Here's how the part is built. I have some questions about the finished solid (model axes, mm). A direction names the side the tool comes from. Coordinates: 2 decimals unless noted, no trailing zeros. Loops run counter-clockwise (first coordinate to the right, second up) from the corner with the lowest first, then second, coordinate; pieces in that order, holes last.
```python
from build123d import *

# Parameters (mm, degrees)
SKETCH1_W           = 15
SKETCH1_H           = 35
BOSS_EXTRUDE1_DEPTH = 5
SKETCH2_R           = 1
SKETCH2_W           = 12
SKETCH2_H           = 22
CUT_EXTRUDE1_DEPTH  = 5
BOSS_EXTRUDE2_DEPTH = 5


with BuildPart() as part:
    # Sketch1 → Boss-Extrude1 (new body)
    with BuildSketch(Plane.XY):
        with Locations((-15.154109589, 0.428082192)):
            Rectangle(SKETCH1_W, SKETCH1_H)
    extrude(amount=BOSS_EXTRUDE1_DEPTH)

    # Sketch2 → Cut-Extrude1 (cut)
    with BuildSketch(Plane.XY.offset(5)):
        with Locations((-15.154109589, -12.571917808)):
            Circle(SKETCH2_R)
        with Locations((-15.154109589, 13.428082192)):
            Circle(SKETCH2_R)
        with Locations((-15.154109589, 0.428082192)):
            Rectangle(SKETCH2_W, SKETCH2_H)
    extrude(amount=-CUT_EXTRUDE1_DEPTH, mode=Mode.SUBTRACT)

    # Sketch3 → Boss-Extrude2 (add)
    with BuildSketch(Plane.XY.offset(5)):
        Polygon((-22.654109589, -17.071917808), (-22.654109589, -30.804233772), (-20.282646179, -47.190952111), (-17.359431797, -56.865022466), (-13.811210888, -68.607486145), (0, -68.607486145), (6.832413717, -38.997592941), (-6.905605444, -30.804233772), (-7.654109589, -17.071917808), align=None)
    extrude(amount=-BOSS_EXTRUDE2_DEPTH)


solid = part.part
```
1. I need wall thicknesses on line 1 along X through (y, z) = (9.5, 2.35); line 2 along Y through (x, z) = (-12.5, 3.75); line 3 along X through (y, z) = (-14, 3.55). Which ranges of each line are inside material? Lowest first, please.
2. I want a section at A-A (y = 7). Please give me the cut outline in (x, z).
3. I want a section at C-C (z = 2.3). Please give me the cut outline in (x, y).
4. On a 3-axis mill with a long thin cutter (end or side, diameter ignored), from which of +Z, -Z, +X, -X, +Y, -Y can I reach the whole of each face in a straight line? I mean faces 1 (the flat face through (-15, 17.928, 2)), 2 (the flat face through (-15, -10.572, 3)), 3 (the flat face through (-7.654, 0, 2)). Say none if no direction works.
5. For pin 1 (1 mm diameter, centred on x = 2.5, z = 3.5, fed in from +Y); pin 2 (1.5 mm diameter, centred on y = 4.5, z = 2.5, fed in from +X), each with a flat end and sliding along its axis, tell me the tip position at first contact or that it passes through.
6. I want a section at B-B (x = -11.5). Please give me the cut outline in (y, z), then the cut area to 3 significant figures.
7. I want a section at D-D (x = -5.75). Please give me the cut outline in (y, z), then the cut area to 3 significant figures.
8. We'd pull the mould along X, two halves only. Please class faces 4 (the flat face through (-15, 11.428, 3)), 5 (the flat face through (-7.275, -24.034, 2.535)), 6 (the flat face through (-22.654, -6, 3)): +X half, -X half, draft (parallel to the pull), parting line (faces both ways), or undercut.
Response values:
1. line 1: x = -22.65 to -21.15, -9.15 to -7.65
1. line 2: y = -68.61 to -10.57, 11.43 to 17.93
1. line 3: x = -22.65 to -7.65
2. outline: (-22.65, 0) - (-21.15, 0) - (-21.15, 5) - (-22.65, 5) - close; (-9.15, 0) - (-7.65, 0) - (-7.65, 5) - (-9.15, 5) - close
3. outline: (-22.65, -30.8) - (-20.28, -47.19) - (-13.81, -68.61) - (0, -68.61) - (6.83, -39) - (-6.91, -30.8) - (-7.65, -17.07) - (-7.65, 17.93) - (-22.65, 17.93) - close; hole (-21.15, -10.57) - (-9.15, -10.57) - (-9.15, 11.43) - (-21.15, 11.43) - close; hole circle Ø2 at (-15.15, -12.57); hole circle Ø2 at (-15.15, 13.43)
4. face 1: +Z, -Z, +X, -X, +Y
4. face 2: +Z, -Z
4. face 3: +Z, -Z, +X, +Y
5. pin 1: stops at y = -36.12
5. pin 2: stops at x = -7.65
6. outline: (-68.61, 0) - (-10.57, 0) - (-10.57, 5) - (-68.61, 5) - close; (11.43, 0) - (17.93, 0) - (17.93, 5) - (11.43, 5) - close
6. area: 323 mm2
7. outline: (-68.61, 0) - (-31.49, 0) - (-31.49, 5) - (-68.61, 5) - close
7. area: 186 mm2
8. face 4: undercut
8. face 5: +X half
8. face 6: -X half
